Work out the finished part from the listing and answer in its coordinate system (mm). A direction names the side the tool comes from. Coordinates: 2 decimals unless noted, no trailing zeros. Order: outer loops, then holes, each group sorted by start corner. A loop starts at its lowest first (then second) coordinate and runs counter-clockwise, first axis right, second up. Notation, with made-up numbers: (46, 11.5) - (64, 11.5) arc R10 cw to (64, 27.5) - close; hole circle Ø5 at (-38, 18.5). An arc over 180 degrees is marked (long way). Use CSV: the item, a comma, the result in double quotes. Start each with the question number.
from build123d import *

# Parameters (mm, degrees)
CROQUIS1_W              = 266
CROQUIS1_H              = 150
CROQUIS1_W_2            = 50
CROQUIS1_H_2            = 6
CROQUIS1_W_3            = 6
CROQUIS1_H_3            = 50
SALIENTE_EXTRUIR1_DEPTH = 6
CROQUIS3_W              = 14
CROQUIS3_H              = 150
SALIENTE_EXTRUIR4_DEPTH = 6


with BuildPart() as part:
    # Croquis1 → Saliente-Extruir1 (new body)
    with BuildSketch(Plane.XY):
        Rectangle(CROQUIS1_W, CROQUIS1_H)
        with Locations((-108, 78)):
            Rectangle(CROQUIS1_W_2, CROQUIS1_H_2)
        with Locations((0, 78)):
            Rectangle(CROQUIS1_W_2, CROQUIS1_H_2)
        with Locations((-108, -78)):
            Rectangle(CROQUIS1_W_2, CROQUIS1_H_2)
        with Locations((0, -78)):
            Rectangle(CROQUIS1_W_2, CROQUIS1_H_2)
        with Locations((108, -78)):
            Rectangle(CROQUIS1_W_2, CROQUIS1_H_2)
        with Locations((-136, 0)):
            Rectangle(CROQUIS1_W_3, CROQUIS1_H_3)
        with Locations((108, 78)):
            Rectangle(CROQUIS1_W_2, CROQUIS1_H_2)
    extrude(amount=SALIENTE_EXTRUIR1_DEPTH)

    # Croquis3 → Saliente-Extruir4 (add)
    with BuildSketch(Plane.XY.offset(6)):
        with Locations((140, 0)):
            Rectangle(CROQUIS3_W, CROQUIS3_H)
    extrude(amount=-SALIENTE_EXTRUIR4_DEPTH)


solid = part.part
1) The part is cut by section B-B on x = 62. Determine the outline of the cut face in (y, z), plus the area to 3 significant figures.
2) Straight lines are drawn through the part: line 1 (Y direction, x = 39.5, z = 5.2); line 2 (X direction, y = 26.5, z = 2.3). For each, find the intervals that lie inside material, in ascending order. Write a range as [from, to].
3) For a pull along X with two mould halves and no side action, classify faces 4 (the face through (140, -75, 3)), 5 (the face through (-139, 0, 3)), 6 (the face through (-25, 78, 3)) as +X half, -X half, draft (parallel to the pull), parting line (faces both ways), or undercut.
4) The part is cut by section C-C on y = -54.5. Determine the outline of the cut face in (x, z).
5) The part is cut by section A-A on z = 2.1. Determine the outline of the cut face in (x, y), plus the area to 3 significant figures.
6) Flat-ended cylindrical pins translate along their axes: P1, Ø1.8, axis at y = 49.5, z = 3, coming from the -X side; P2, Ø1.8, axis at x = 138.5, z = 2.5, coming from the -Y side; P3, Ø3, axis at x = 142.5, z = 3, coming from the +Y side. Find the tip coordinate at first contact, or state that the pin passes through.
7) For faces 1 (the face through (-136, 25, 3)), 2 (the face through (-54, 75, 3)), 3 (the face through (133, -78, 3)), determine the directions among +Z, -Z, +X, -X, +Y, -Y from which every point of the face is accessible in a straight line to the end or side of a thin tool.
Answer key:
1,outline,"(-75, 0) - (75, 0) - (75, 6) - (-75, 6) - close"
1,area,"900 mm^2"
2,line 1,"[-75, 75]"
2,line 2,"[-133, 147]"
3,face 4,"draft"
3,face 5,"-X half"
3,face 6,"undercut"
4,outline,"(-133, 0) - (147, 0) - (147, 6) - (-133, 6) - close"
5,outline,"(-139, -25) - (-133, -25) - (-133, -81) - (-83, -81) - (-83, -75) - (-25, -75) - (-25, -81) - (25, -81) - (25, -75) - (83, -75) - (83, -81) - (133, -81) - (133, -75) - (147, -75) - (147, 75) - (133, 75) - (133, 81) - (83, 81) - (83, 75) - (25, 75) - (25, 81) - (-25, 81) - (-25, 75) - (-83, 75) - (-83, 81) - (-133, 81) - (-133, 25) - (-139, 25) - close"
5,area,"44,100 mm^2"
6,P1,"x = -133"
6,P2,"y = -75"
6,P3,"y = 75"
7,face 1,"+Z, -Z, -X, +Y"
7,face 2,"+Z, -Z, +Y"
7,face 3,"+Z, -Z, +X, -Y"
